Here's how the part is built. I have some questions about the finished solid (model axes, mm). A direction names the side the tool comes from. Give positions to 0.01 mm unless a question says otherwise; leave off trailing zeros. Loops run counter-clockwise (first coordinate to the right, second up) from the corner with the lowest first, then second, coordinate; pieces in that order, holes last.
Q1. If we section it at D-D (x = -163): Please give me the cut outline in (y, z).
Q2. If we section it at C-C (y = 154): Please give me the cut outline in (x, z), plus the area to 3 significant figures.
Q3. I need wall thicknesses on line 1 (Y direction, x = -63, z = -784); line 2 (X direction, y = 105.5, z = -889); line 3 (X direction, y = 73, z = -146.5). Which ranges of each line are inside material? Lowest first, please.
Q4. For faces 1 (the face through (-192.2, 2.5, -103)), 2 (the face through (-4.5, 33.3, -203.2)), 3 (the face through (-11.43, 60, -895)), 4 (the face through (-57, 5.08, -1017)), which set-ups out of +Z, -Z, +X, -X, +Y, -Y let a thin tool reach every point of the face, with its end or its side?
Q5. If we section it at B-B (z = -165): Please give me the cut outline in (x, y).
Q6. If we section it at A-A (y = 56): Please give me the cut outline in (x, z), plus the area to 3 significant figures.
Q7. Will these pins go through, and if not, where does the flat tip stop? P1, Ø3, axis at x = -10, z = -1077, coming from the +Y side; P2, Ø8, axis at x = -67, z = -1253.5, coming from the -Y side; P3, Ø4, axis at x = -23, z = -1859.5, coming from the +Y side.
Q8. We'd pull the mould along Z, two halves only. Please class faces 5 (the face through (-163, 5.08, -69)), 6 (the face through (-5.08, 55, -1017)), 7 (the face through (-44, 52, -1866.9)), 8 (the face through (-34, 5, 38.1)): +Z half, -Z half, draft (parallel to the pull), parting line (faces both ways), or undercut.
from build123d import *

# Parameters (mm, degrees)
F1_DEPTH = 38.1
F6_DEPTH = 1905
F7_W     = 279.4
F7_H     = 279.4
F8_DEPTH = 12.7


with BuildPart() as f1:
    # F0 (on Top) → F1 (new body)
    with BuildSketch(Plane.XY):
        Polygon((-254, 0), (0, 0), (0, 254), (-5.08, 254), (-5.08, 5.08), (-254, 5.08), align=None)
    extrude(amount=F1_DEPTH)

    # F1_face (on face) → F4 section 0
    with BuildSketch(Plane(origin=(-65.398586, 65.398586, 0), x_dir=(1, 0, 0), z_dir=(0, 0, -1))):
        Polygon((65.398586, 65.398586), (-188.601414, 65.398586), (-188.601414, 60.318586), (60.318586, 60.318586), (60.318586, -188.601414), (65.398586, -188.601414), align=None)
    # F3 (on offset) → F4 section 1
    with BuildSketch(Plane.XY.offset(-203.2)):
        Polygon((-132.08, 0), (0, 0), (0, 132.08), (-5.08, 132.08), (-5.08, 5.08), (-132.08, 5.08), align=None)
    loft()

    # F5 (on face) → F6 (join)
    with BuildSketch(Plane.XY.offset(38.1)):
        Polygon((-106.68, 5.08), (-5.08, 5.08), (-5.08, 106.68), (-11.43, 106.68), (-11.43, 11.43), (-106.68, 11.43), align=None)
    extrude(amount=-F6_DEPTH)

    # F7 (on face) → F8 (join)
    with BuildSketch(Plane(origin=(0, 0, -1866.9), x_dir=(1, 0, 0), z_dir=(0, 0, -1))):
        with Locations((-42.072112, -54.21998)):
            Rectangle(F7_W, F7_H)
    extrude(amount=-F8_DEPTH)


solid = f1.part
Check sheet entries:
1. outline: (-85.48, -1866.9) - (193.92, -1866.9) - (193.92, -1854.2) - (-85.48, -1854.2) - close; (0, -151.67) - (5.08, -151.67) - (5.08, 38.1) - (0, 38.1) - close
2. outline: (-181.77, -1866.9) - (97.63, -1866.9) - (97.63, -1854.2) - (-181.77, -1854.2) - close; (-5.08, -166.67) - (0, -166.67) - (0, 38.1) - (-5.08, 38.1) - close
2. area: 4,590 mm2
3. line 1: y = 5.08 to 11.43
3. line 2: x = -11.43 to -5.08
3. line 3: x = -11.43 to 0
4. face 1: -X, +Y, -Y
4. face 2: +X, -Y
4. face 3: +Z, -X, +Y
4. face 4: +X, -X, -Y
5. outline: (-155, 0) - (0, 0) - (0, 155) - (-5.08, 155) - (-5.08, 106.68) - (-11.43, 106.68) - (-11.43, 11.43) - (-106.68, 11.43) - (-106.68, 5.08) - (-155, 5.08) - close
6. outline: (-181.77, -1866.9) - (97.63, -1866.9) - (97.63, -1854.2) - (-5.08, -1854.2) - (-5.08, -203.2) - (0, -203.2) - (0, 38.1) - (-11.43, 38.1) - (-11.43, -1854.2) - (-181.77, -1854.2) - close
6. area: 16,800 mm2
7. P1: stops at y = 106.68
7. P2: stops at y = 5.08
7. P3: stops at y = 193.92
8. face 5: draft
8. face 6: undercut
8. face 7: -Z half
8. face 8: +Z half
